Design review of the part built by this model. Coordinates are the model's own, in mm. Face numbers are marked on the shaded views. A direction names the side the tool comes from. Round coordinates to 2 decimals unless told otherwise and drop trailing zeros. Loops run counter-clockwise (first coordinate to the right, second up) from the corner with the lowest first, then second, coordinate; pieces in that order, holes last. Notation, with made-up numbers: (-20.75, 78) - (-0.75, 78) arc R25 ccw to (-0.75, 108) - close; hole circle Ø10 at (-31.75, 72). An arc over 180 degrees is marked (long way). One line per question, with ' | ' between items. Start each with the question number.
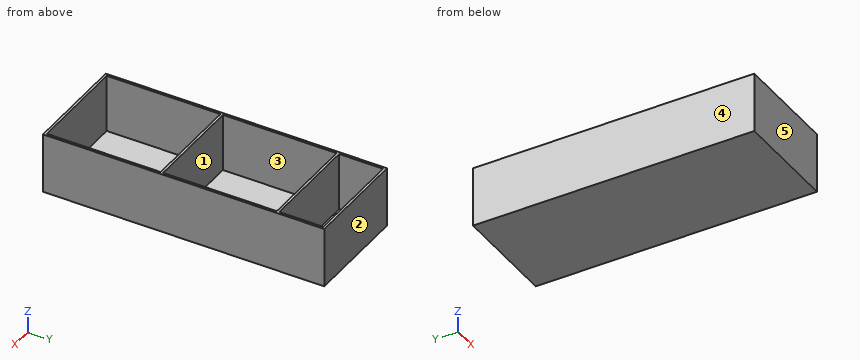
from build123d import *

# Parameters (mm, degrees)
F0_W     = 43.8
F0_H     = 115.8
F1_DEPTH = 24.8
F2_W     = 41.8
F2_H     = 18.133333
F2_H_2   = 46.833334
F2_H_3   = 46.833333
F3_DEPTH = 23.8


with BuildPart() as f1:
    # F0 (on Top) → F1 (new body)
    with BuildSketch(Plane.XY):
        with Locations((21.9, -57.9)):
            Rectangle(F0_W, F0_H)
    extrude(amount=F1_DEPTH)

    # F2 (on face) → F3 (cut)
    with BuildSketch(Plane.XY.offset(24.8)):
        with Locations((21.9, -10.066667)):
            Rectangle(F2_W, F2_H)
        with Locations((21.9, -43.55)):
            Rectangle(F2_W, F2_H_2)
        with Locations((21.9, -91.383333)):
            Rectangle(F2_W, F2_H_3)
    extrude(amount=-F3_DEPTH, mode=Mode.SUBTRACT)


solid = f1.part
1. Take a section at A-A, the plane x = 32. Give the boundary of the cut face in (y, z), then the cut area to 3 significant figures.
2. To check wall thickness, follow line 1 along Y through (x, z) = (15.5, 5.25); line 2 along X through (y, z) = (-105.5, 19.5); line 3 along Z through (x, y) = (22.5, -79). State the ranges of each line that lie inside material, in increasing order.
3. Take a section at B-B, the plane z = 7.75. Give the boundary of the cut face in (x, y).
4. The part is to be moulded in two halves that separate along Y. For the marked faces 3, 4 and 5, say which applies: pulls with the +Y half, pulls with the -Y half, needs draft (parallel to the pull), parting line crosses it, or undercut.
5. Machinability: for the marked faces 1 and 2, which of the approach directions +Z, -Z, +X, -X, +Y, -Y give a long, thin tool a straight path to every point of the face, cutting with its end or side? Answer none if there is none.
6. Clearance check with flat-ended pins moving along their axes: P1, Ø14.5, axis at y = -13, z = 9, coming from the -X side; P2, Ø9, axis at x = 32, y = -6, coming from the +Z side. State where each tip first meets the part, or that it passes through.
7. Take a section at C-C, the plane y = -75. Give the boundary of the cut face in (x, z), then the cut area to 3 significant figures.
Answer list:
1) outline: (-115.8, 0) - (0, 0) - (0, 24.8) - (-1, 24.8) - (-1, 1) - (-19.13, 1) - (-19.13, 24.8) - (-20.13, 24.8) - (-20.13, 1) - (-66.97, 1) - (-66.97, 24.8) - (-67.97, 24.8) - (-67.97, 1) - (-114.8, 1) - (-114.8, 24.8) - (-115.8, 24.8) - close | area: 211 mm²
2) line 1: y = -115.8 to -114.8, -67.97 to -66.97, -20.13 to -19.13, -1 to 0 | line 2: x = 0 to 1, 42.8 to 43.8 | line 3: z = 0 to 1
3) outline: (0, -115.8) - (43.8, -115.8) - (43.8, 0) - (0, 0) - close; hole (1, -114.8) - (42.8, -114.8) - (42.8, -67.97) - (1, -67.97) - close; hole (1, -66.97) - (42.8, -66.97) - (42.8, -20.13) - (1, -20.13) - close; hole (1, -19.13) - (42.8, -19.13) - (42.8, -1) - (1, -1) - close
4) face 3: undercut | face 4: needs draft | face 5: pulls with the -Y half
5) face 1: +Z | face 2: +Z, -Z, +X, -X, +Y
6) P1: stops at x = 0 | P2: stops at z = 1
7) outline: (0, 0) - (43.8, 0) - (43.8, 24.8) - (42.8, 24.8) - (42.8, 1) - (1, 1) - (1, 24.8) - (0, 24.8) - close | area: 91.4 mm²
